Here's how the part is built. I have some questions about the finished solid (model axes, mm). A direction names the side the tool comes from. Coordinates: 2 decimals unless noted, no trailing zeros. Write each loop counter-clockwise with the first axis right and the second up, starting at its lowest first coordinate (ties: lowest second). Pieces come first, ordered by that corner, then holes. Notation, with made-up numbers: M -9.75,57 L 48.25,57 A30 cw 48.25,87 Z; hole C 33,-13 d9. An arc over 180 degrees is marked long. Use a Markdown table: item, result.
```python
from build123d import *

# Parameters (mm, degrees)
SKETCH3_W           = 72.39
SKETCH3_H           = 26.67
BOSS_EXTRUDE1_DEPTH = 12.7
SKETCH4_R           = 16.002
CUT_EXTRUDE1_DEPTH  = 26.4
SKETCH7_R           = 3.3782
CUT_EXTRUDE2_DEPTH  = 15.875
FILLET1_R           = 2.54
CUT_EXTRUDE3_DEPTH  = 4.064


with BuildPart() as part:
    # Sketch3 → Boss-Extrude1 (new body, symmetric)
    with BuildSketch(Plane.XY):
        Rectangle(SKETCH3_W, SKETCH3_H)
    extrude(amount=BOSS_EXTRUDE1_DEPTH, both=True)

    # Sketch4 → Cut-Extrude1 (cut, through all)
    with BuildSketch(Plane.XY.offset(12.7)):
        with Locations((0, -13.335)):
            Circle(SKETCH4_R)
    extrude(amount=-CUT_EXTRUDE1_DEPTH, mode=Mode.SUBTRACT)

    # Sketch7 → Cut-Extrude2 (cut, symmetric)
    with BuildSketch(Plane(origin=(0, 0, 0), x_dir=(1, 0, 0), z_dir=(0, 1, 0))):
        with Locations((-26.101920205, 0)):
            Circle(SKETCH7_R)
    cut_extrude2 = extrude(amount=CUT_EXTRUDE2_DEPTH, both=True, mode=Mode.SUBTRACT)

    # Mirror1: Cut-Extrude2 across plane
    add(cut_extrude2.mirror(Plane(origin=(0, 0, 0), x_dir=(0, 0, 1), z_dir=(1, 0, 0))), mode=Mode.SUBTRACT)

    # Fillet1
    fillet1_edges = [part.edges().sort_by_distance(p)[0] for p in [
        (36.195, 0, 12.7),
        (0, 13.335, -12.7),
        (36.195, 0, -12.7),
        (-36.195, 13.335, 0),
        (36.195, 13.335, 0),
        (0, 13.335, 12.7),
    ]]
    fillet(fillet1_edges, radius=FILLET1_R)

    # Sketch8 → Cut-Extrude3 (cut)
    with BuildSketch(Plane(origin=(0, 13.335, 0), x_dir=(1, 0, 0), z_dir=(0, 1, 0))):
        Polygon((-26.101920205, -6.599113577), (-20.386920205, -3.299556788), (-20.386920205, 3.299556788), (-26.101920205, 6.599113577), (-31.816920205, 3.299556788), (-31.816920205, -3.299556788), align=None)
    cut_extrude3 = extrude(amount=-CUT_EXTRUDE3_DEPTH, mode=Mode.SUBTRACT)

    # Mirror2: Cut-Extrude3 across plane
    add(cut_extrude3.mirror(Plane(origin=(0, 0, 0), x_dir=(0, 0, 1), z_dir=(1, 0, 0))), mode=Mode.SUBTRACT)


solid = part.part
```
1. Will this pin go through, and if not, where does the flat tip stop? pin 1 Ø2 at (y, z) = (12, 1.5) entering from -X.
Answers follow:
| item | result |
|---|---|
| pin 1 | stops at x = -36.19 |
2. We'd pull the mould along X, two halves only. Please class faces 3 (the face through (-28.92, 11.33, -4.97)), 4 (the face through (36.195, -1, 0)), 5 (the face through (-2, 4, -12.7)): +X half, -X half, draft (parallel to the pull), parting line (faces both ways), or undercut.
Answers follow:
| item | result |
|---|---|
| face 3 | undercut |
| face 4 | +X half |
| face 5 | draft |
3. Suppose I cut it at A-A on z = 0. Write out the boundary of the cut face in (x, y) (3 decimals).
Answers follow:
| item | result |
|---|---|
| outline | M -36.195,-13.335 L -29.48,-13.335 L -29.48,9.271 L -31.817,9.271 L -31.817,13.335 L -33.655,13.335 A2.54 ccw -36.195,10.795 Z; M -22.724,-13.335 L -16.002,-13.335 A16.002 cw 16.002,-13.335 L 22.724,-13.335 L 22.724,9.271 L 20.387,9.271 L 20.387,13.335 L -20.387,13.335 L -20.387,9.271 L -22.724,9.271 Z; M 29.48,-13.335 L 36.195,-13.335 L 36.195,10.795 A2.54 ccw 33.655,13.335 L 31.817,13.335 L 31.817,9.271 L 29.48,9.271 Z |
4. Suppose I cut it at D-D on y = -3.5. Write out the boundary of the cut face in (x, z) (3 decimals), and give its area (3 significant figures).
Answers follow:
| item | result |
|---|---|
| outline | M -36.195,-12.7 L -12.623,-12.7 L -12.623,12.7 L -36.195,12.7 Z; M 12.623,-12.7 L 33.655,-12.7 A2.54 ccw 36.195,-10.16 L 36.195,10.16 A2.54 ccw 33.655,12.7 L 12.623,12.7 Z; hole C -26.102,0 d6.756; hole C 26.102,0 d6.756 |
| area | 1,120 mm2 |
5. Suppose I cut it at B-B on y = -11. Write out the boundary of the cut face in (x, z) (3 decimals).
Answers follow:
| item | result |
|---|---|
| outline | M -36.195,-12.7 L -15.831,-12.7 L -15.831,12.7 L -36.195,12.7 Z; M 15.831,-12.7 L 33.655,-12.7 A2.54 ccw 36.195,-10.16 L 36.195,10.16 A2.54 ccw 33.655,12.7 L 15.831,12.7 Z; hole C -26.102,0 d6.756; hole C 26.102,0 d6.756 |
6. I need wall thicknesses on probe 1 along X at (y, z) = (10.5, 5.5) (3 decimals); probe 2 along X at (y, z) = (9.5, 6) (3 decimals); probe 3 along Z at (x, y) = (-23, 2). Which ranges of each line are inside material? Lowest first, please.
Answers follow:
| item | result |
|---|---|
| probe 1 | x = -36.195 to -28.006, -24.198 to 24.198, 28.006 to 36.195 |
| probe 2 | x = -36.195 to -27.14, -25.064 to 25.064, 27.14 to 36.195 |
| probe 3 | z = -12.7 to -1.34, 1.34 to 12.7 |
7. Suppose I cut it at C-C on x = 0. Write out the boundary of the cut face in (y, z) (3 decimals).
Answers follow:
| item | result |
|---|---|
| outline | M 2.667,-12.7 L 10.795,-12.7 A2.54 ccw 13.335,-10.16 L 13.335,10.16 A2.54 ccw 10.795,12.7 L 2.667,12.7 Z |
8. Which directions (+Z, -Z, +X, -X, +Y, -Y) give clear straight access to the entire face, cutting with the end or side of a thin tool? Please do faces 1 (the face through (-23.28, 11.33, 4.97)), 2 (the face through (-36.195, -1, 0)).
Answers follow:
| item | result |
|---|---|
| face 1 | +Y |
| face 2 | +Z, -Z, -X, +Y, -Y |
